from build123d import *

# Parameters (mm, degrees)
SKETCH1_W           = 232.477284974
SKETCH1_H           = 16.858001952
BOSS_EXTRUDE1_DEPTH = 100
SKETCH2_R           = 25
BOSS_EXTRUDE2_DEPTH = 70
SKETCH5_R           = 20
BOSS_EXTRUDE3_DEPTH = 20
BOSS_EXTRUDE3_TAPER = 13
SKETCH6_R           = 15.382636177
BOSS_EXTRUDE4_DEPTH = 80
SKETCH7_R           = 15.382636177
BOSS_EXTRUDE5_DEPTH = 20
BOSS_EXTRUDE5_TAPER = 36
LPATTERN1_COUNT     = 2
LPATTERN1_PITCH     = 80
LPATTERN2_COUNT     = 2
LPATTERN2_PITCH     = 80
SKETCH9_R           = 120
BOSS_EXTRUDE6_DEPTH = 250
BOSS_EXTRUDE6_DRAFT = -20.8


with BuildPart() as part:
    # Sketch1 → Boss-Extrude1 (new body)
    with BuildSketch(Plane.XY):
        Rectangle(SKETCH1_W, SKETCH1_H)
    extrude(amount=BOSS_EXTRUDE1_DEPTH)

    # Sketch2 → Boss-Extrude2 (add)
    with BuildSketch(Plane(origin=(0, 8.429000976, 0), x_dir=(1, 0, 0), z_dir=(0, 1, 0))):
        with Locations(Location((0, -50, 0), (0, 0, 270))):
            Circle(SKETCH2_R)
    extrude(amount=BOSS_EXTRUDE2_DEPTH)

    # Sketch5 → Boss-Extrude3 (add)
    with BuildSketch(Plane.XZ.offset(8.429000976)):
        with Locations((0, 50)):
            Circle(SKETCH5_R)
    boss_extrude3 = extrude(amount=BOSS_EXTRUDE3_DEPTH, taper=BOSS_EXTRUDE3_TAPER)

    # Sketch6 → Boss-Extrude4 (add)
    with BuildSketch(Plane.XZ.offset(28.429000976)):
        with Locations(Location((0, 50, 0), (0, 0, 270))):
            Circle(SKETCH6_R)
    boss_extrude4 = extrude(amount=BOSS_EXTRUDE4_DEPTH)

    # Sketch7 → Boss-Extrude5 (add)
    with BuildSketch(Plane.XZ.offset(108.429000976)):
        with Locations(Location((0, 50, 0), (0, 0, 270))):
            Circle(SKETCH7_R)
    boss_extrude5 = extrude(amount=BOSS_EXTRUDE5_DEPTH, taper=BOSS_EXTRUDE5_TAPER)

    # LPattern1: Boss-Extrude3, Boss-Extrude4, Boss-Extrude5 ×2
    with Locations(*[(i * LPATTERN1_PITCH, 0, 0) for i in range(1, LPATTERN1_COUNT)]):
        add(boss_extrude3)
        add(boss_extrude4)
        add(boss_extrude5)

    # LPattern2: Boss-Extrude3, Boss-Extrude4, Boss-Extrude5 ×2
    with Locations(*[(-i * LPATTERN2_PITCH, 0, 0) for i in range(1, LPATTERN2_COUNT)]):
        add(boss_extrude3)
        add(boss_extrude4)
        add(boss_extrude5)


with BuildPart() as boss_extrude6_tool:
    # Sketch9 → Boss-Extrude6 (with draft: the straight prism first)
    with BuildSketch(Plane(origin=(0, 328.429000976, 0), x_dir=(1, 0, 0), z_dir=(0, 1, 0))):
        with Locations((0, -50)):
            Circle(SKETCH9_R)
    extrude(amount=-BOSS_EXTRUDE6_DEPTH)
    # Boss-Extrude6: the draft: its side faces are tilted about the plane it starts from
    boss_extrude6_sides = [boss_extrude6_tool.faces().sort_by_distance(p)[0] for p in [
        (-120, 203.429000976, 50),
    ]]
    draft(boss_extrude6_sides, Plane(origin=(0, 328.429000976, 0), x_dir=(1, 0, 0), z_dir=(0, 1, 0)), BOSS_EXTRUDE6_DRAFT)


with BuildPart() as part_1:
    add(part.part)

    # Boss-Extrude6: add boss_extrude6_tool
    add(boss_extrude6_tool.part)


solid = part_1.part
Here's how the part is built. I have some questions about the finished solid (model axes, mm). A direction names the side the tool comes from. Round coordinates to 2 decimals unless told otherwise and drop trailing zeros. Loops run counter-clockwise (first coordinate to the right, second up) from the corner with the lowest first, then second, coordinate; pieces in that order, holes last.
1. For P1, Ø8.5, axis at x = 38, y = 1, coming from the +Z side; P2, Ø18.5, axis at y = -1.5, z = 67.5, coming from the +X side; P3, Ø3, axis at y = 208.5, z = 2, coming from the -X side, each with a flat end and sliding along its axis, tell me the tip position at first contact or that it passes through.
Answer list:
P1: stops at z = 100
P2: stops at x = 116.24
P3: stops at x = -58.34
2. Which directions (+Z, -Z, +X, -X, +Y, -Y) give clear straight access to the entire face, cutting with the end or side of a thin tool? Please do faces 4 (the face through (70.64, -67.869, 62.207)), 5 (the face through (-2, 0, 0)), 6 (the face through (-2, 0, 100)).
Answer list:
face 4: -Y
face 5: -Z, +X, -X, -Y
face 6: +Z, +X, -X, -Y
3. We'd pull the mould along X, two halves only. Please class faces 1 (the face through (0.676, -67.869, 65.368)), 2 (the face through (-2, 328.429, 48)), 3 (the face through (-116.239, 0, 49)): +X half, -X half, draft (parallel to the pull), parting line (faces both ways), or undercut.
Answer list:
face 1: undercut
face 2: draft
face 3: -X half
4. If I drill on line 1 along Z through (x, y) = (22, 156.5); line 2 along Y through (x, z) = (33.5, 14.5); line 3 along X through (y, z) = (-14.5, 50), over which ranges is the centre line in solid material (lowest first)?
Answer list:
line 1: z = -0.07 to 100.07
line 2: y = -8.43 to 8.43, 141.02 to 328.43
line 3: x = -98.6 to -61.4, -18.6 to 18.6, 61.4 to 98.6
5. If we section it at A-A on y = -70: Write out the boundary of the cut face in (x, z).
Answer list:
outline: circle Ø30.77 at (-80, 50); circle Ø30.77 at (0, 50); circle Ø30.77 at (80, 50)
6. If we section it at B-B on y = 205.5: Write out the boundary of the cut face in (x, z), plus the area to 3 significant figures.
Answer list:
outline: circle Ø146.61 at (0, 50)
area: 16,900 mm2
